```python
from build123d import *

# Parameters (mm, degrees)
ESBO_O1_W                 = 170
ESBO_O1_H                 = 30
ESBO_O1_R                 = 5
ESBO_O1_R_2               = 3.5
ESBO_O1_R_3               = 2
RESSALTO_EXTRUS_O1_DEPTH  = 10
CORTE_EXTRUS_O1_START     = 26.451612903
CORTE_EXTRUS_O1_OUTLINE_R = 1.5
CORTE_EXTRUS_O1_DEPTH     = 30


# Read off the part's stored shape, not the designer's step: Corte-extrusão1
with BuildPart() as part:
    # Esboço1 → Ressalto-extrusão1 (new body)
    with BuildSketch(Plane.XY):
        with Locations((-192.217741935, 41.451612903)):
            Rectangle(ESBO_O1_W, ESBO_O1_H)
        with Locations((-192.217741935, 41.451612903)):
            Circle(ESBO_O1_R, mode=Mode.SUBTRACT)
        with Locations((-242.217741935, 41.451612903)):
            Circle(ESBO_O1_R_2, mode=Mode.SUBTRACT)
        with Locations((-142.217741935, 41.451612903)):
            Circle(ESBO_O1_R_2, mode=Mode.SUBTRACT)
        with Locations((-257.217741935, 41.451612903)):
            Circle(ESBO_O1_R_3, mode=Mode.SUBTRACT)
        with Locations((-127.217741935, 41.451612903)):
            Circle(ESBO_O1_R_3, mode=Mode.SUBTRACT)
    extrude(amount=RESSALTO_EXTRUS_O1_DEPTH)

    # Corte-extrusão1 outline → Corte-extrusão1 (cut)
    with BuildSketch(Plane(origin=(0, 0, 0), x_dir=(1, 0, 0), z_dir=(0, 1, 0)).offset(CORTE_EXTRUS_O1_START)):
        with Locations((-210.23272287, -4.918113723)):
            Circle(CORTE_EXTRUS_O1_OUTLINE_R)
        with Locations((-176.768107745, -4.912217988)):
            Circle(CORTE_EXTRUS_O1_OUTLINE_R)
    extrude(amount=CORTE_EXTRUS_O1_DEPTH, mode=Mode.SUBTRACT)


solid = part.part
```
Source: CAD feature listing. Evaluate the final solid. Frame: model axes, mm. Give positions to 0.01 mm unless a question says otherwise; leave off trailing zeros. Loops run counter-clockwise (first coordinate to the right, second up) from the corner with the lowest first, then second, coordinate; pieces in that order, holes last. Notation, with made-up numbers: (45.25, -7.5) -> (64.25, -7.5) arc R10 ccw to (64.25, 6.5) -> close; hole circle Ø8 at (-22, -10). An arc over 180 degrees is marked (long way). Put each result on its own line as item: value. Start each with the question number.
1) Cut plane B-B (z = 1.5). Return loops of the section in (x, y), then the cut area to 3 significant figures.
2) Draft query along X for faces 1 (the face through (-277.218, 41, 5)), 2 (the face through (-259.216, 41.54, 4.93)), 3 (the face through (-193, 48, 0)). Return one class per face: released by +X, released by -X, zero draft, split by the parting line, or undercut.
3) Contact query for a flat-ended pin moving along its axis: P1, Ø2.5, axis at x = -127.22, y = 41.45, coming from the -Z side. Output: stop coordinate, or through.
4) Material intervals for probe 1 along Y at (x, z) = (-257, 7.25); probe 2 along X at (y, z) = (33.5, 5.5); probe 3 along X at (y, z) = (43.5, 6.5), sorted ascending.
5) Cut plane A-A (x = -242.5). Return loops of the section in (y, z), then the cut area to 3 significant figures.
6) Cut plane C-C (x = -191.5). Return loops of the section in (y, z).
Results are:
1. outline: (-277.22, 26.45) -> (-107.22, 26.45) -> (-107.22, 56.45) -> (-277.22, 56.45) -> close; hole circle Ø4 at (-257.22, 41.45); hole circle Ø7 at (-242.22, 41.45); hole circle Ø10 at (-192.22, 41.45); hole circle Ø7 at (-142.22, 41.45); hole circle Ø4 at (-127.22, 41.45)
1. area: 4,920 mm2
2. face 1: released by -X
2. face 2: undercut
2. face 3: zero draft
3. P1: passes through
4. probe 1: y = 26.45 to 39.46, 43.44 to 56.45
4. probe 2: x = -277.22 to -211.62, -208.85 to -178.15, -175.39 to -107.22
4. probe 3: x = -277.22 to -245.06, -239.38 to -196.78, -187.66 to -145.06, -139.38 to -107.22
5. outline: (26.45, 0) -> (37.96, 0) -> (37.96, 10) -> (26.45, 10) -> close; (44.94, 0) -> (56.45, 0) -> (56.45, 10) -> (44.94, 10) -> close
5. area: 230 mm2
6. outline: (26.45, 0) -> (36.5, 0) -> (36.5, 10) -> (26.45, 10) -> close; (46.4, 0) -> (56.45, 0) -> (56.45, 10) -> (46.4, 10) -> close
